from build123d import *

# Parameters (mm, degrees)
BOSS_EXTRUDE1_DEPTH = 13
SKETCH2_W           = 8.229441325
SKETCH2_H           = 8
CUT_EXTRUDE1_DEPTH  = 100
FILLET1_R           = 1


with BuildPart() as part:
    # Sketch1 → Boss-Extrude1 (new body)
    with BuildSketch(Plane.XY):
        Polygon((0, 0), (40, 0), (40, 51), (33, 51), (33, 3), (0, 3), align=None)
    extrude(amount=BOSS_EXTRUDE1_DEPTH)

    # Sketch2 → Cut-Extrude1 (cut)
    with BuildSketch(Plane(origin=(40, 0, 0), x_dir=(0, 0, -1), z_dir=(1, 0, 0))):
        Polygon((-3, 39), (-13, 39), (-13, 0), (-10, 0), (-10, 3), (-3, 3), align=None)
        with Locations((-7.114720663, 45)):
            Rectangle(SKETCH2_W, SKETCH2_H)
    extrude(amount=-CUT_EXTRUDE1_DEPTH, mode=Mode.SUBTRACT)

    # Mirror2: part across plane


with BuildPart() as part_1:
    add(part.part)
    add(part.part.mirror(Plane(origin=(0, 0, 13), x_dir=(0, 0, 1), z_dir=(1, 0, 0))))

    # Fillet1
    fillet1_edges = [part_1.edges().sort_by_distance(p)[0] for p in [
        (-40, 0, 5),
        (0, 0, 10),
        (40, 0, 5),
        (40, 1.5, 10),
        (40, 41, 7.114720663),
        (40, 45, 11.229441325),
        (40, 49, 7.114720663),
        (40, 45, 3),
        (33, 45, 3),
        (33, 3, 1.5),
        (33, 49, 7.114720663),
        (33, 45, 11.229441325),
        (33, 41, 7.114720663),
        (36.5, 3, 3),
        (0, 3, 10),
        (-36.5, 3, 3),
        (-33, 3, 1.5),
        (-33, 45, 3),
        (-33, 49, 7.114720663),
        (-33, 45, 11.229441325),
        (-33, 41, 7.114720663),
        (-40, 41, 7.114720663),
        (-40, 45, 11.229441325),
        (-40, 49, 7.114720663),
        (-40, 45, 3),
        (-36.5, 51, 0),
        (-36.5, 51, 13),
        (-36.5, 39, 13),
        (-36.5, 39, 3),
        (36.5, 39, 3),
        (36.5, 39, 13),
        (36.5, 51, 13),
        (36.5, 51, 0),
        (-40, 1.5, 10),
    ]]
    fillet(fillet1_edges, radius=FILLET1_R)


solid = part_1.part
CAD build for the part. Positions are in the model's coordinates, mm. A direction names the side the tool comes from. Give positions to 0.01 mm unless a question says otherwise; leave off trailing zeros. Order: outer loops, then holes, each group sorted by start corner. A loop starts at its lowest first (then second) coordinate and runs counter-clockwise, first axis right, second up. Notation, with made-up numbers: (55.5, 59) - (59.5, 59) arc R33 cw to (59.5, 88) - close; hole circle Ø6 at (-13, 23.5). An arc over 180 degrees is marked (long way). Answer in a Markdown table with one row per item.
1. Saw through at B-B, the plane y = 28. Give the cut face in (x, z), plus the area to 3 significant figures.
Data:
| item | result |
|---|---|
| outline | (-40, 0) - (-33, 0) - (-33, 3) - (-40, 3) - close; (33, 0) - (40, 0) - (40, 3) - (33, 3) - close |
| area | 42.0 mm² |
2. Saw through at A-A, the plane z = 6.5. Count the separate pieces of the cut face and the enclosed holes in it, plus the area to 3 significant figures.
Data:
| item | result |
|---|---|
| separate pieces | 5 |
| enclosed holes | 0 |
| area | 294 mm² |
3. Probe probe 1 along Y at (x, z) = (13, 7.5); probe 2 along X at (y, z) = (36.5, 1.75); probe 3 along Z at (x, y) = (-24, 2). List the from-to ranges inside material, lowest first. Write a range as [from, to].
Data:
| item | result |
|---|---|
| probe 1 | y = [0, 3] |
| probe 2 | x = [-40, -33], [33, 40] |
| probe 3 | z = [0, 10] |
4. Flat gauge pins, fed straight in: pin 1 (1.1 mm diameter, centred on x = 10, y = 1.5, fed in from +Z); pin 2 (1.5 mm diameter, centred on x = 23.5, z = 9.5, fed in from +Y); pin 3 (2 mm diameter, centred on x = -38, y = 16.5, fed in from +Z). Where does each tip first touch, or does it go through?
Data:
| item | result |
|---|---|
| pin 1 | stops at z = 10 |
| pin 2 | stops at y = 3 |
| pin 3 | stops at z = 3 |
5. Tool access for faces 4 (the flat face through (33, 31, 2)), 5 (the flat face through (36, 45, 13)), 6 (the flat face through (-37, 39, 8)), 7 (the flat face through (-1, 3, 4)), 8 (the flat face through (-37, 45, 3)): list every direction of +Z, -Z, +X, -X, +Y, -Y with a clear straight run to the whole face (end or side of a thin tool).
Data:
| item | result |
|---|---|
| face 4 | +Z, -Z, +Y |
| face 5 | +Z, +X, -X, +Y, -Y |
| face 6 | +Z, +X, -X |
| face 7 | +Z |
| face 8 | +X, -X |
6. Saw through at C-C, the plane x = 25.5. Give the cut face in (y, z), plus the area to 3 significant figures.
Data:
| item | result |
|---|---|
| outline | (0, 0) - (3, 0) - (3, 9) arc R1 ccw to (2, 10) - (1, 10) arc R1 ccw to (0, 9) - close |
| area | 29.6 mm² |
7. Pull direction Z, two halves, no side cores. Call faces 1 (the flat face through (37, 21, 3)), 2 (the flat face through (-37, 51, 6)), 3 (the flat face through (37, 41, 7)): pulls with the +Z half, pulls with the -Z half, needs draft (parallel to the pull), parting line crosses it, or undercut.
Data:
| item | result |
|---|---|
| face 1 | pulls with the +Z half |
| face 2 | needs draft |
| face 3 | undercut |
